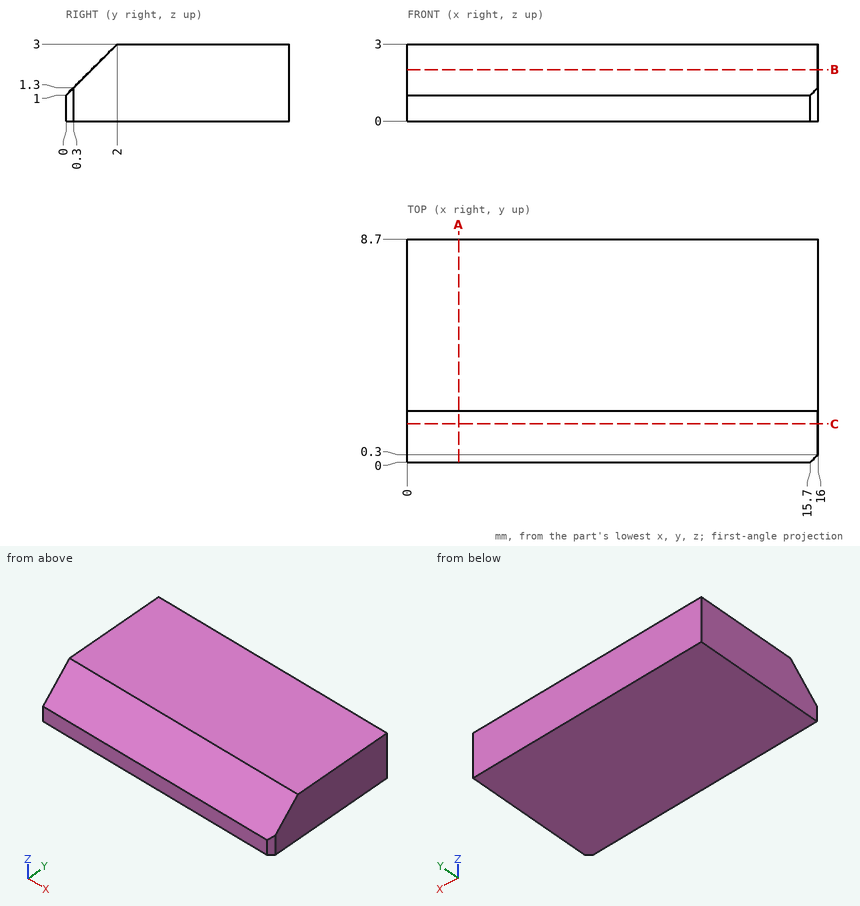
The drawing under review shows one solid part. Ordinate dimensions are in mm from its lowest x, y, z. Coordinates: 2 decimals unless noted, no trailing zeros. Write each loop counter-clockwise with the first axis right and the second up, starting at its lowest first coordinate (ties: lowest second). Pieces come first, ordered by that corner, then holes. Notation, with made-up numbers: (-21, 61.5) -> (33, 61.5) arc R16 ccw to (33, 71.5) -> close; hole circle Ø9 at (-29, 81.25). An arc over 180 degrees is marked (long way). Write each question's results on one line, items separated by ' | '. Start each with the question number.
1) Insertion check: pin 1 (1 mm diameter, centred on x = 8, z = 2, fed in from -Y). The pin has a flat end and moves straight along its axis. Give the tip position at first contact, or say it passes through.
2) Consider section C-C (y = 1.5). Write out the cut boundary in (x, z), plus the area to 3 significant figures.
3) Wall thickness on L1, parallel to Y at x = 4.25, z = 1.3; L2, parallel to Y at x = 11.5, z = 2.4; L3, parallel to Z at x = 9.75, y = 1.75: over which ranges is each line inside the solid? List them lowest first. Write a range as [from, to].
4) Consider section B-B (z = 2). Write out the cut boundary in (x, y), plus the area to 3 significant figures.
5) Consider section A-A (x = 2). Write out the cut boundary in (y, z).
Geometry says:
1) pin 1: y = 0.5
2) outline: (0, 0) -> (16, 0) -> (16, 2.5) -> (0, 2.5) -> close | area: 40.0 mm^2
3) L1: [0.3, 8.7] | L2: [1.4, 8.7] | L3: [0, 2.75]
4) outline: (0, 1) -> (16, 1) -> (16, 8.7) -> (0, 8.7) -> close | area: 123 mm^2
5) outline: (0, 0) -> (8.7, 0) -> (8.7, 3) -> (2, 3) -> (0, 1) -> close
